Geometry: see drawing. Coordinates: mm, zero at the bounding-box minimum. A direction names the side the tool comes from. Give positions to 0.01 mm unless a question says otherwise; leave off trailing zeros. Loops run counter-clockwise (first coordinate to the right, second up) from the corner with the lowest first, then second, coordinate; pieces in that order, holes last. Notation, with made-up numbers: (-24.75, 85) -> (17.25, 85) arc R22 ccw to (17.25, 105) -> close; hole circle Ø7 at (4, 13.5). An arc over 180 degrees is marked (long way). Use CSV: the item, a comma, the result in double quotes.
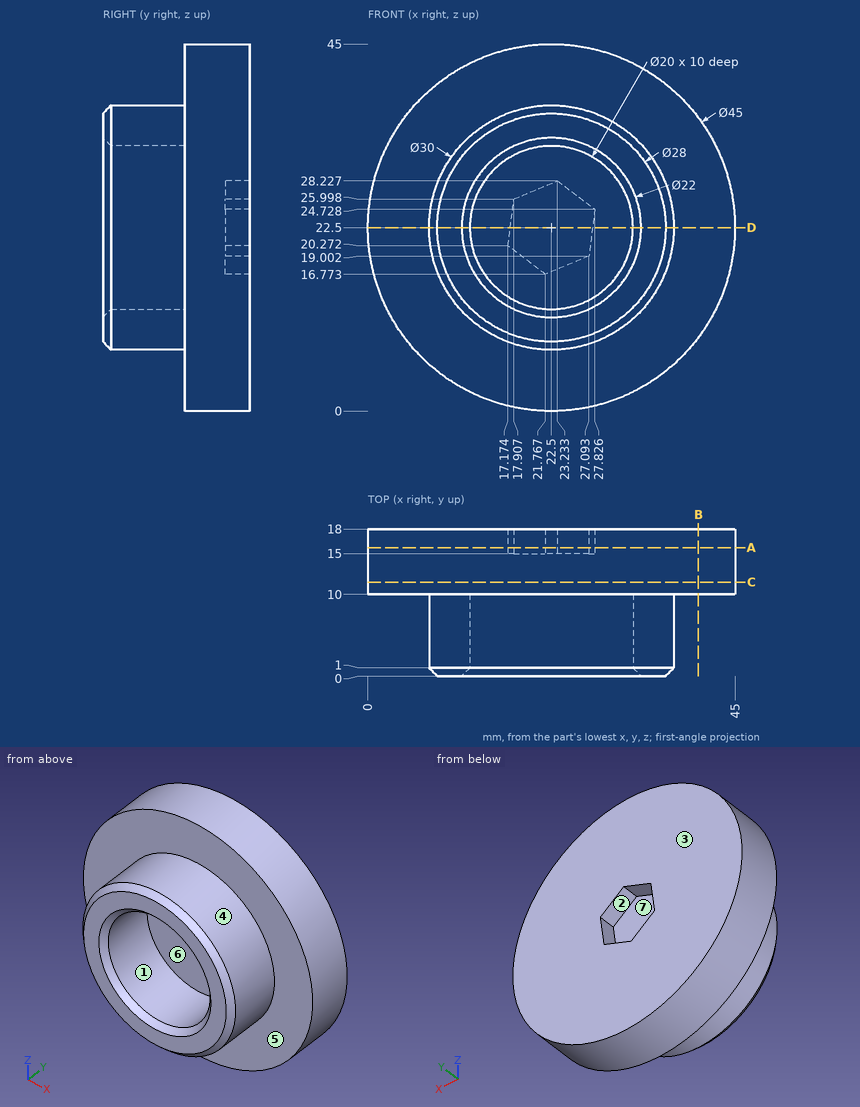
1) Ray query, line 1 (X direction, y = 6.25, z = 22.5); line 2 (Y direction, x = 39.5, z = 30.5); line 3 (Z direction, x = 25, y = 17) (1 decimal). Return the intervals inside material, ascending.
From the geometry:
line 1,"x = 7.5 to 12.5, 32.5 to 37.5"
line 2,"y = 10 to 18"
line 3,"z = 0.1 to 18.1, 26.9 to 44.9"
2) Section query C-C (y = 11.5). Return loops of the section in (x, z).
From the geometry:
outline,"circle Ø45 at (22.5, 22.5)"
3) Contact query for flat-ended pins moving along their axis: pin 1 (8 mm diameter, centred on x = 10, z = 39.5, fed in from -Y); pin 2 (4 mm diameter, centred on x = 25.5, z = 15, fed in from -Y); pin 3 (1 mm diameter, centred on x = 24, z = 25, fed in from +Y). Output: stop coordinate, or through.
From the geometry:
pin 1,"stops at y = 10"
pin 2,"stops at y = 0.92"
pin 3,"stops at y = 15"
4) Section query D-D (z = 22.5). Return loops of the section in (x, y), then the cut area to 3 significant figures.
From the geometry:
outline,"(0, 10) -> (7.5, 10) -> (7.5, 1) -> (8.5, 0) -> (11.5, 0) -> (12.5, 1) -> (12.5, 10) -> (32.5, 10) -> (32.5, 1) -> (33.5, 0) -> (36.5, 0) -> (37.5, 1) -> (37.5, 10) -> (45, 10) -> (45, 18) -> (27.54, 18) -> (27.54, 15) -> (17.46, 15) -> (17.46, 18) -> (0, 18) -> close"
area,"428 mm^2"
5) Section query A-A (y = 15.75). Return loops of the section in (x, z), then the cut area to 3 significant figures.
From the geometry:
outline,"circle Ø45 at (22.5, 22.5); hole (17.17, 20.27) -> (21.77, 16.77) -> (27.09, 19) -> (27.83, 24.73) -> (23.23, 28.23) -> (17.91, 26) -> close"
area,"1,500 mm^2"
6) Section query B-B (x = 40.5). Return loops of the section in (y, z), then the cut area to 3 significant figures.
From the geometry:
outline,"(10, 9) -> (18, 9) -> (18, 36) -> (10, 36) -> close"
area,"216 mm^2"
7) Mould query, pull axis X, two halves, no side actions, for the marked faces 4, 5, 6 and 7. Classes: pulls with the +X half, pulls with the -X half, needs draft (parallel to the pull), parting line crosses it, or undercut.
From the geometry:
face 4,"parting line crosses it"
face 5,"needs draft"
face 6,"undercut"
face 7,"undercut"
8) Reachability of the marked faces 1, 2 and 3 from +Z, -Z, +X, -X, +Y, -Y: full face, straight path, thin tool, end or side. Return the list, or none.
From the geometry:
face 1,"-Y"
face 2,"+Y"
face 3,"+Z, -Z, +X, -X, +Y"
